The listing builds one solid part. Answer for the finished solid, in the listing's coordinates (mm). A direction names the side the tool comes from. Round coordinates to 2 decimals unless told otherwise and drop trailing zeros. Loops run counter-clockwise (first coordinate to the right, second up) from the corner with the lowest first, then second, coordinate; pieces in that order, holes last. Notation, with made-up numbers: (71, 36.25) - (94, 36.25) arc R20 cw to (94, 69.25) - close; hole circle Ø2 at (-37.5, 19.5). An arc over 180 degrees is marked (long way). One line per item, written item: value.
```python
from build123d import *

# Parameters (mm, degrees)
PAD_DEPTH       = 11
SKETCH001_R     = 3.25
POCKET_DEPTH    = 6
SKETCH002_R     = 3.25
POCKET001_DEPTH = 6
FILLET_R        = 1


with BuildPart() as part:
    # Sketch → Pad (new body, symmetric)
    with BuildSketch(Plane.YZ):
        Polygon((-60, 0), (0, 0), (-42.4264068712, 42.4264068712), (-46.6690475583, 38.1837661841), (-31.1022907321, 22.6170093579), (-37.9852813742, 6), (-60, 6), align=None)
        Polygon((-28.627416998, 20.1421356237), (-34.4852813742, 6), (-14.4852813742, 6), align=None, mode=Mode.SUBTRACT)
    extrude(amount=PAD_DEPTH, both=True)

    # Sketch001 (on Face6 of Pad) → Pocket (cut)
    with BuildSketch(Plane(origin=(0, 0, 6), x_dir=(0, -1, 0), z_dir=(0, 0, 1))):
        with Locations((50, 0)):
            Circle(SKETCH001_R)
    extrude(amount=-POCKET_DEPTH, mode=Mode.SUBTRACT)

    # Sketch002 (on Face9 of Pocket) → Pocket001 (cut)
    with BuildSketch(Plane(origin=(0, -4.2426406871, -4.2426406871), x_dir=(0, 0.7071067812, -0.7071067812), z_dir=(0, -0.7071067812, -0.7071067812))):
        with Locations((-50, 0)):
            Circle(SKETCH002_R)
    extrude(amount=-POCKET001_DEPTH, mode=Mode.SUBTRACT)

    # Fillet
    fillet_edges = [part.edges().sort_by_distance(p)[0] for p in [
        (0, 0, 0),
        (0, -60, 0),
        (0, -60, 6),
        (0, -46.669048, 38.183766),
        (0, -42.426407, 42.426407),
    ]]
    fillet(fillet_edges, radius=FILLET_R)


solid = part.part
```
1) A cutting plane is placed at C-C on x = 0. Give the vertices of the cut face in (y, z).
Final values:
outline: (-60, 1) arc R1 ccw to (-59, 0) - (-53.25, 0) - (-53.25, 6) - (-59, 6) arc R1 ccw to (-60, 5) - close; (-46.75, 0) - (-2.41, 0) arc R1 ccw to (-1.71, 1.71) - (-33.06, 33.06) - (-37.3, 28.81) - (-31.1, 22.62) - (-37.99, 6) - (-46.75, 6) - close; (-45.96, 37.48) - (-41.9, 33.41) - (-37.65, 37.65) - (-41.72, 41.72) arc R1 ccw to (-43.13, 41.72) - (-45.96, 38.89) arc R1 ccw to start; hole (-34.49, 6) - (-14.49, 6) - (-28.63, 20.14) - close
2) Consider L1, parallel to X at y = -50, z = 3; L2, parallel to Z at x = -2.75, y = -34; L3, parallel to Z at x = 7.75, y = -23. Determine where each line is inside the solid, lowest interval first.
Final values:
L1: -11 to -3.25, 3.25 to 11
L2: 0 to 6, 7.17 to 15.62, 25.51 to 34
L3: 0 to 6, 14.51 to 23
3) For a pull along Z with two mould halves and no side action, classify faces 1 (the flat face through (0.15, -44.53, 40.32)), 2 (the flat face through (0.154, -21.457, 12.972)), 3 (the flat face through (11, -33, 12)) as released by +Z, released by -Z, zero draft, split by the parting line, or undercut.
Final values:
face 1: released by +Z
face 2: undercut
face 3: zero draft
4) A cutting plane is placed at D-D on z = 16. Give the vertices of the cut face in (x, y), and give its area (3 significant figures).
Final values:
outline: (-11, -33.84) - (11, -33.84) - (11, -30.34) - (-11, -30.34) - close; (-11, -24.49) - (11, -24.49) - (11, -16) - (-11, -16) - close
area: 264 mm2
5) Each of these flat-tipped pins is pushed along its axis until it touches: pin 1 Ø10.5 at (x, y) = (-3, -45) entering from +Z; pin 2 Ø1 at (x, z) = (-4.5, 19.5) entering from -Y; pin 3 Ø5 at (x, y) = (0, -50) entering from -Z; pin 4 Ø1 at (x, z) = (3.5, 25.5) entering from -Y. Where does it stop, or does it pass through?
Final values:
pin 1: z = 42.01
pin 2: y = -32.6
pin 3: through
pin 4: y = -34.49
6) A cutting plane is placed at A-A on y = -50. Give the vertices of the cut face in (x, z), and give its area (3 significant figures).
Final values:
outline: (-11, 0) - (-3.25, 0) - (-3.25, 6) - (-11, 6) - close; (3.25, 0) - (11, 0) - (11, 6) - (3.25, 6) - close
area: 93.0 mm2
7) A cutting plane is placed at B-B on x = -8. Give the vertices of the cut face in (y, z).
Final values:
outline: (-60, 1) arc R1 ccw to (-59, 0) - (-2.41, 0) arc R1 ccw to (-1.71, 1.71) - (-41.72, 41.72) arc R1 ccw to (-43.13, 41.72) - (-45.96, 38.89) arc R1 ccw to (-45.96, 37.48) - (-31.1, 22.62) - (-37.99, 6) - (-59, 6) arc R1 ccw to (-60, 5) - close; hole (-34.49, 6) - (-14.49, 6) - (-28.63, 20.14) - close
8) For faces 4 (the flat face through (0, -60, 3)), 5 (the flat face through (0, -46, 6)), 6 (the flat face through (0.154, -31.515, 13.17)), determine the directions among +Z, -Z, +X, -X, +Y, -Y from which every point of the face is accessible in a straight line to the end or side of a thin tool.
Final values:
face 4: +Z, -Z, +X, -X, -Y
face 5: +X, -X, -Y
face 6: +X, -X
